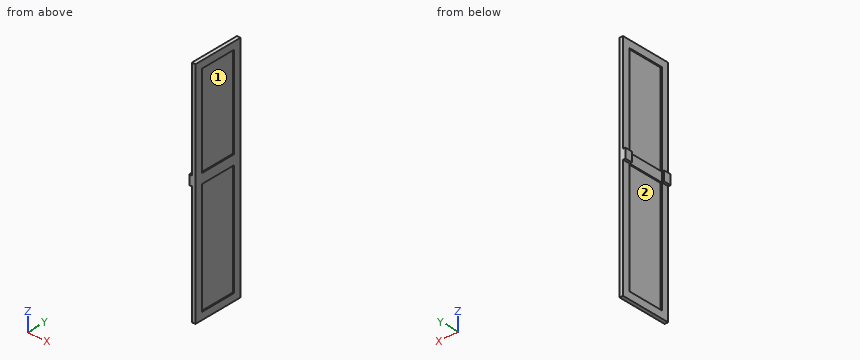
from build123d import *

# Parameters (mm, degrees)
F0_W     = 425
F0_H     = 1900
F1_DEPTH = 30
F2_W     = 305
F2_H     = 764.579544
F2_H_2   = 935.420456
F3_DEPTH = 10
F4_W     = 305
F4_H     = 764.579544
F4_H_2   = 935.420456
F5_DEPTH = 10
F6_W     = 60
F6_H     = 80
F7_DEPTH = 20


with BuildPart() as f1:
    # F0 (on Right) → F1 (new body)
    with BuildSketch(Plane.YZ):
        with Locations((212.5, 950)):
            Rectangle(F0_W, F0_H)
    extrude(amount=F1_DEPTH)

    # F2 (on face) → F3 (cut)
    with BuildSketch(Plane.YZ.offset(30)):
        with Locations((212.5, 1457.710228)):
            Rectangle(F2_W, F2_H)
        with Locations((212.5, 527.710228)):
            Rectangle(F2_W, F2_H_2)
    extrude(amount=-F3_DEPTH, mode=Mode.SUBTRACT)

    # F4 (on face) → F5 (cut)
    with BuildSketch(Plane(origin=(0, 0, 0), x_dir=(0, -1, 0), z_dir=(-1, 0, 0))):
        with Locations((-212.5, 1457.710228)):
            Rectangle(F4_W, F4_H)
        with Locations((-212.5, 527.710228)):
            Rectangle(F4_W, F4_H_2)
    extrude(amount=-F5_DEPTH, mode=Mode.SUBTRACT)

    # F6 (on face) → F7 (join)
    with BuildSketch(Plane(origin=(0, 0, 0), x_dir=(0, -1, 0), z_dir=(-1, 0, 0))):
        with Locations((-395, 1035.420456)):
            Rectangle(F6_W, F6_H)
        with Locations((-30, 1035.420456)):
            Rectangle(F6_W, F6_H)
    extrude(amount=F7_DEPTH)


solid = f1.part
Input: part model. Units: mm. Frame: model coordinates. Face numbers are marked on the shaded views. A direction names the side the tool comes from. Give positions to 0.01 mm unless a question says otherwise; leave off trailing zeros. Loops run counter-clockwise (first coordinate to the right, second up) from the corner with the lowest first, then second, coordinate; pieces in that order, holes last. Notation, with made-up numbers: (75.25, -4.5) - (103.25, -4.5) arc R18 ccw to (103.25, 2.5) - close; hole circle Ø4 at (32, -24.75). An arc over 180 degrees is marked (long way). Use CSV: the item, a comma, the result in double quotes. Start each with the question number.
Item 1: Section B-B on y = 394.5. Return loops of the section in (x, z), then the cut area to 3 significant figures.
Item 2: Reachability of the marked faces 1 and 2 from +Z, -Z, +X, -X, +Y, -Y: full face, straight path, thin tool, end or side. Return the list, or none.
Item 3: Section D-D on y = 206. Return loops of the section in (x, z).
Item 4: Line query: line 1 (Z direction, x = 27, y = 251); line 2 (Y direction, x = 26.5, z = 525.5); line 3 (X direction, y = 48.5, z = 1171.5). Output: solid intervals per line, ascending.
Item 5: Contact query for flat-ended pins moving along their axis: P1, Ø16, axis at x = -14, y = 404.5, coming from the -Z side; P2, Ø5, axis at y = 300.5, z = 1522, coming from the -X side; P3, Ø2, axis at y = 211.5, z = 694, coming from the +X side. Output: stop coordinate, or through.
Item 6: Section C-C on z = 954.5. Return loops of the section in (x, y).
Item 7: Section A-A on x = -8. Return loops of the section in (y, z), then the cut area to 3 significant figures.
Ans:
1,outline,"(-20, 995.42) - (0, 995.42) - (0, 0) - (30, 0) - (30, 1900) - (0, 1900) - (0, 1075.42) - (-20, 1075.42) - close"
1,area,"58,600 mm2"
2,face 1,"+X"
2,face 2,"-X"
3,outline,"(0, 0) - (30, 0) - (30, 60) - (20, 60) - (20, 995.42) - (30, 995.42) - (30, 1075.42) - (20, 1075.42) - (20, 1840) - (30, 1840) - (30, 1900) - (0, 1900) - (0, 1840) - (10, 1840) - (10, 1075.42) - (0, 1075.42) - (0, 995.42) - (10, 995.42) - (10, 60) - (0, 60) - close"
4,line 1,"z = 0 to 60, 995.42 to 1075.42, 1840 to 1900"
4,line 2,"y = 0 to 60, 365 to 425"
4,line 3,"x = 0 to 30"
5,P1,"stops at z = 995.42"
5,P2,"stops at x = 10"
5,P3,"stops at x = 20"
6,outline,"(0, 0) - (30, 0) - (30, 60) - (20, 60) - (20, 365) - (30, 365) - (30, 425) - (0, 425) - (0, 365) - (10, 365) - (10, 60) - (0, 60) - close"
7,outline,"(0, 995.42) - (60, 995.42) - (60, 1075.42) - (0, 1075.42) - close; (365, 995.42) - (425, 995.42) - (425, 1075.42) - (365, 1075.42) - close"
7,area,"9,600 mm2"
